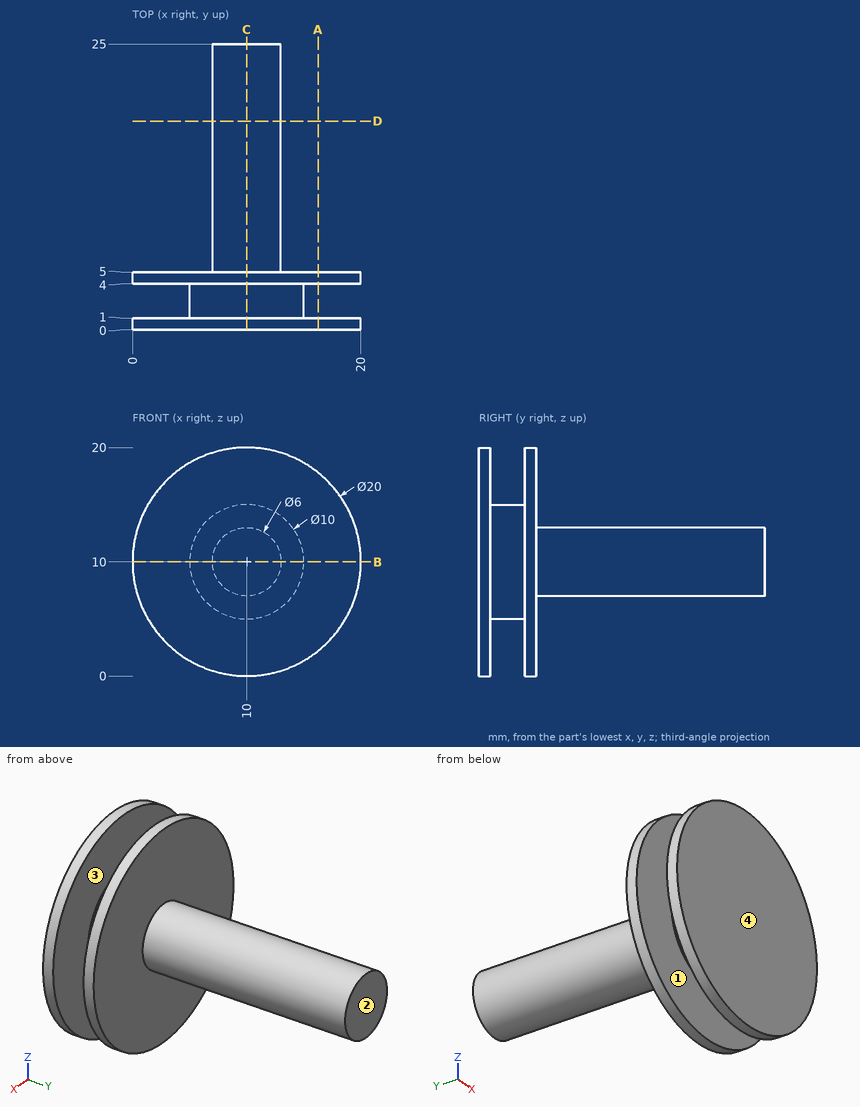
Input: dimensioned drawing with shaded views. Units: mm. Origin: part minimum x, y, z. Coordinates: 2 decimals unless noted, no trailing zeros. Order: outer loops, then holes, each group sorted by start corner. A loop starts at its lowest first (then second) coordinate and runs counter-clockwise, first axis right, second up.
(1) Section query B-B (z = 10). Return the cut outline in (x, y).
(2) First-contact query: pin 1 (10 mm diameter, centred on x = 13, y = 16.5, fed in from +Z); pin 2 (3 mm diameter, centred on y = 12.5, z = 8, fed in from +X); pin 3 (10 mm diameter, centred on y = 22.5, z = 8, fed in from -X); pin 4 (3 mm diameter, centred on x = 16.5, z = 17, fed in from -Y). Flat tips, straight axial feed; report the tip coordinate or a pass-through.
(3) Section query C-C (x = 10). Return the cut outline in (y, z), plus the area to 3 significant figures.
(4) Section query D-D (y = 18.25). Return the cut outline in (x, z), plus the area to 3 significant figures.
(5) Draft query along Y for the marked faces 1, 2, 3 and 4. Return one class per face: pulls with the +Y half, pulls with the -Y half, needs draft (parallel to the pull), parting line crosses it, or undercut.
(6) Material intervals for probe 1 along Y at (x, z) = (16.25, 8); probe 2 along Z at (x, y) = (10, 12); probe 3 along Y at (x, z) = (6.5, 10.25), sorted ascending.
(7) Section query A-A (x = 16.25). Return the cut outline in (y, z), plus the area to 3 significant figures.
Solution:
1. outline: (0, 0) - (20, 0) - (20, 1) - (15, 1) - (15, 4) - (20, 4) - (20, 5) - (13, 5) - (13, 25) - (7, 25) - (7, 5) - (0, 5) - (0, 4) - (5, 4) - (5, 1) - (0, 1) - close
2. pin 1: stops at z = 13
2. pin 2: stops at x = 12.96
2. pin 3: stops at x = 7
2. pin 4: stops at y = 0
3. outline: (0, 0) - (1, 0) - (1, 5) - (4, 5) - (4, 0) - (5, 0) - (5, 7) - (25, 7) - (25, 13) - (5, 13) - (5, 20) - (4, 20) - (4, 15) - (1, 15) - (1, 20) - (0, 20) - close
3. area: 190 mm2
4. outline: circle Ø6 at (10, 10)
4. area: 28.3 mm2
5. face 1: undercut
5. face 2: pulls with the +Y half
5. face 3: undercut
5. face 4: pulls with the -Y half
6. probe 1: y = 0 to 1, 4 to 5
6. probe 2: z = 7 to 13
6. probe 3: y = 0 to 5
7. outline: (0, 2.19) - (1, 2.19) - (1, 17.81) - (0, 17.81) - close; (4, 2.19) - (5, 2.19) - (5, 17.81) - (4, 17.81) - close
7. area: 31.2 mm2
